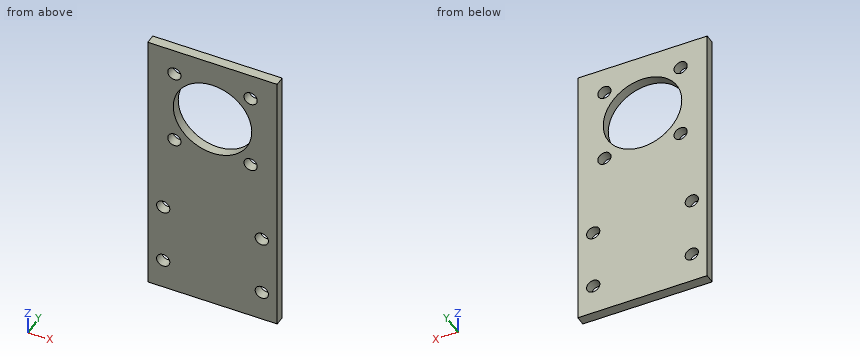
from build123d import *

# Parameters (mm, degrees)
SKETCH1_W            = 42
SKETCH1_H            = 90
SKETCH1_R            = 12.75
BOSS_EXTRUDE1_DEPTH  = 3.175
M4_CLEARANCE_HOLE1_D = 4.3


with BuildPart() as part:
    # Sketch1 → Boss-Extrude1 (new body)
    with BuildSketch(Plane(origin=(0, 0, 0), x_dir=(1, 0, 0), z_dir=(0, 1, 0))):
        with Locations((21, 45)):
            Rectangle(SKETCH1_W, SKETCH1_H)
        with Locations(Location((21, 21, 0), (0, 0, 270))):
            Circle(SKETCH1_R, mode=Mode.SUBTRACT)
    extrude(amount=BOSS_EXTRUDE1_DEPTH)

    # M4 Clearance Hole1 (through all)
    with Locations(Plane(origin=(0, 3.175, 0), x_dir=(1, 0, 0), z_dir=(0, 1, 0))):
        with Locations((8.625631329, 33.374368671), (21, 21), (5, 80), (33.374368671, 33.374368671), (33.374368671, 8.625631329), (8.625631329, 8.625631329), (37, 80), (37, 60), (5, 60)):
            Hole(M4_CLEARANCE_HOLE1_D / 2)


solid = part.part
Model file for the job. Use its own axes, mm. Give positions to 0.01 mm unless a question says otherwise; leave off trailing zeros. Write each loop counter-clockwise with the first axis right and the second up, starting at its lowest first coordinate (ties: lowest second). Pieces come first, ordered by that corner, then holes. Notation, with made-up numbers: M -29.5,31 L -12.5,31 A20 ccw -12.5,66 Z; hole C 13,-4.75 d1. An arc over 180 degrees is marked long. One line per item, written item: value. Start each with the question number.
Q1. Saw through at D-D, the plane y = 1.95. State how many separate pieces and enclosed holes the cut face has, plus the area to 3 significant figures.
Q2. Probe probe 1 along X at (y, z) = (1.05, -80); probe 2 along Z at (x, y) = (20.5, 2.9); probe 3 along Z at (x, y) = (37.5, 1.8). List the from-to ranges inside material, lowest first. Write a range as [from, to].
Q3. Saw through at C-C, the plane z = -80. Write the cut outline in (x, y) (3 decimals), plus the area to 3 significant figures.
Q4. Saw through at B-B, the plane x = 5. Write the cut outline in (y, z) (3 decimals).
Q5. Saw through at A-A, the plane z = -21. Write the cut outline in (x, y) (3 decimals).
Output values:
1. separate pieces: 1
1. enclosed holes: 9
1. area: 3,150 mm²
2. probe 1: x = [0, 2.85], [7.15, 34.85], [39.15, 42]
2. probe 2: z = [-90, -33.74], [-8.26, 0]
2. probe 3: z = [-90, -82.09], [-77.91, -62.09], [-57.91, 0]
3. outline: M 0,0 L 2.85,0 L 2.85,3.175 L 0,3.175 Z; M 7.15,0 L 34.85,0 L 34.85,3.175 L 7.15,3.175 Z; M 39.15,0 L 42,0 L 42,3.175 L 39.15,3.175 Z
3. area: 106 mm²
4. outline: M 0,-90 L 3.175,-90 L 3.175,-82.15 L 0,-82.15 Z; M 0,-77.85 L 3.175,-77.85 L 3.175,-62.15 L 0,-62.15 Z; M 0,-57.85 L 3.175,-57.85 L 3.175,0 L 0,0 Z
5. outline: M 0,0 L 8.25,0 L 8.25,3.175 L 0,3.175 Z; M 33.75,0 L 42,0 L 42,3.175 L 33.75,3.175 Z
